```python
from build123d import *

# Parameters (mm, degrees)
BOSS_EXTRUDE1_DEPTH  = 4.7625
M4_CLEARANCE_HOLE1_D = 4.5


with BuildPart() as part:
    # Sketch1 → Boss-Extrude1 (new body)
    with BuildSketch(Plane.XY):
        with BuildLine():
            Line((288.228651321, -1867.207577199), (284.343172474, -1871.093056046))
            ThreePointArc((284.343172474, -1871.093056046), (283.201800398, -1870.89932849), (282.045921758, -1870.834481355))
            Line((282.045921758, -1870.834481355), (248.429921758, -1870.834481355))
            Line((248.429921758, -1870.834481355), (248.429921758, -1866.924781355))
            ThreePointArc((248.429921758, -1866.924781355), (242.929921758, -1861.424781355), (237.429921758, -1866.924781355))
            Line((237.429921758, -1866.924781355), (237.429921758, -1870.834481355))
            Line((237.429921758, -1870.834481355), (203.813921758, -1870.834481355))
            ThreePointArc((203.813921758, -1870.834481355), (202.658043118, -1870.89932849), (201.516671043, -1871.093056046))
            Line((201.516671043, -1871.093056046), (197.631192196, -1867.207577199))
            ThreePointArc((197.631192196, -1867.207577199), (189.853017603, -1867.207577199), (189.853017603, -1874.985751792))
            Line((189.853017603, -1874.985751792), (193.73849645, -1878.871230639))
            ThreePointArc((193.73849645, -1878.871230639), (193.544768893, -1880.012602715), (193.479921758, -1881.168481355))
            Line((193.479921758, -1881.168481355), (193.479921758, -1911.609481355))
            Line((193.479921758, -1911.609481355), (189.570221758, -1911.609481355))
            ThreePointArc((189.570221758, -1911.609481355), (184.070221758, -1917.109481355), (189.570221758, -1922.609481355))
            Line((189.570221758, -1922.609481355), (193.479921758, -1922.609481355))
            Line((193.479921758, -1922.609481355), (193.479921758, -1953.050481355))
            ThreePointArc((193.479921758, -1953.050481355), (193.544768893, -1954.206359995), (193.73849645, -1955.347732071))
            Line((193.73849645, -1955.347732071), (189.853017603, -1959.233210918))
            ThreePointArc((189.853017603, -1959.233210918), (189.853017603, -1967.011385511), (197.631192196, -1967.011385511))
            Line((197.631192196, -1967.011385511), (201.516671043, -1963.125906664))
            ThreePointArc((201.516671043, -1963.125906664), (202.658043118, -1963.31963422), (203.813921758, -1963.384481355))
            Line((203.813921758, -1963.384481355), (282.045921758, -1963.384481355))
            ThreePointArc((282.045921758, -1963.384481355), (283.201800398, -1963.31963422), (284.343172474, -1963.125906664))
            Line((284.343172474, -1963.125906664), (288.228651321, -1967.011385511))
            ThreePointArc((288.228651321, -1967.011385511), (296.006825914, -1967.011385511), (296.006825914, -1959.233210918))
            Line((296.006825914, -1959.233210918), (292.121347067, -1955.347732071))
            ThreePointArc((292.121347067, -1955.347732071), (292.315074623, -1954.206359995), (292.379921758, -1953.050481355))
            Line((292.379921758, -1953.050481355), (292.379921758, -1922.609481355))
            Line((292.379921758, -1922.609481355), (296.289621758, -1922.609481355))
            ThreePointArc((296.289621758, -1922.609481355), (301.789621758, -1917.109481355), (296.289621758, -1911.609481355))
            Line((296.289621758, -1911.609481355), (292.379921758, -1911.609481355))
            Line((292.379921758, -1911.609481355), (292.379921758, -1881.168481355))
            ThreePointArc((292.379921758, -1881.168481355), (292.315074623, -1880.012602715), (292.121347067, -1878.871230639))
            Line((292.121347067, -1878.871230639), (296.006825914, -1874.985751792))
            ThreePointArc((296.006825914, -1874.985751792), (296.006825914, -1867.207577199), (288.228651321, -1867.207577199))
        make_face()
    extrude(amount=BOSS_EXTRUDE1_DEPTH)

    # M4 Clearance Hole1 (through all)
    with Locations(Plane.XY.offset(4.7625)):
        with Locations((193.742104899, -1963.122298214), (189.570221758, -1917.109481355), (193.742104899, -1871.096664496), (242.929921758, -1866.924781355), (292.117738617, -1871.096664496), (296.289621758, -1917.109481355), (292.117738617, -1963.122298214)):
            Hole(M4_CLEARANCE_HOLE1_D / 2)


solid = part.part
```
Here's how the part is built. I have some questions about the finished solid (model axes, mm). A direction names the side the tool comes from. Round coordinates to 2 decimals unless told otherwise and drop trailing zeros. Order: outer loops, then holes, each group sorted by start corner. A loop starts at its lowest first (then second) coordinate and runs counter-clockwise, first axis right, second up. Notation, with made-up numbers: M 40,9.25 L 89,9.25 A15 cw 89,33.25 Z; hole C 4.25,86.25 d9. An arc over 180 degrees is marked long. Use CSV: the item, a comma, the result in double quotes.
1) I want a section at A-A (y = -1941). List the corners of the cut face in (x, z) for me, then the cut area to 3 significant figures.
Taken from the geometry:
outline,"M 193.48,0 L 292.38,0 L 292.38,4.76 L 193.48,4.76 Z"
area,"471 mm^2"
2) I want a section at B-B (x = 261). List the corners of the cut face in (y, z) for me, then the cut area to 3 significant figures.
Taken from the geometry:
outline,"M -1963.38,0 L -1870.83,0 L -1870.83,4.76 L -1963.38,4.76 Z"
area,"441 mm^2"
3) On a 3-axis mill with a long thin cutter (end or side, diameter ignored), from which of +Z, -Z, +X, -X, +Y, -Y can I reach the whole of each face in a straight line? I mean faces 4 (the cylindrical face through (189.768, -1966.925, 2.348)), 5 (the flat face through (192, -1911.609, 2)), 6 (the flat face through (286.313, -1869.123, 2.348)), 7 (the flat face through (294, -1911.609, 2)). Say none if no direction works.
Taken from the geometry:
face 4,"+Z, -Z"
face 5,"+Z, -Z, -X"
face 6,"+Z, -Z, +Y"
face 7,"+Z, -Z, +X"
4) I need wall thicknesses on line 1 along Y through (x, z) = (296, 3.5); line 2 along X through (y, z) = (-1872.5, 2.3); line 3 along X through (y, z) = (-1953, 4.5). Which ranges of each line are inside material? Lowest first, please. Write a range as [from, to].
Taken from the geometry:
line 1,"[-1967.02, -1959.23], [-1922.61, -1919.34], [-1914.88, -1911.61], [-1874.99, -1867.2]"
line 2,"[188.42, 191.98], [195.5, 290.36], [293.88, 297.44]"
line 3,"[193.48, 292.38]"
5) I'm going to push flat-ended pins straight in: P1, Ø2.5, axis at x = 252.5, z = 1.5, coming from the -Y side; P2, Ø1.2, axis at x = 293.5, z = 3.5, coming from the -Y side; P3, Ø1, axis at y = -1887, z = 3.5, coming from the -X side; P4, Ø4, axis at x = 193.74, y = -1963.12, coming from the +Z side (3 decimals). Where does each tip first touch, or does it pass through?
Taken from the geometry:
P1,"y = -1963.38"
P2,"y = -1968.57"
P3,"x = 193.48"
P4,"through"
6) I want a section at C-C (z = 3.75). Count the separate pieces of the cut face and the enclosed holes in it, then the cut area to 3 significant figures.
Taken from the geometry:
separate pieces,"1"
enclosed holes,"7"
area,"9,610 mm^2"
7) If we mould it in two halves opening along Y, with no side actions, what happens to faces 1 (the cylindrical face through (184.07, -1916.99, 2.35)), 2 (the flat face through (248.43, -1869, 2)), 3 (the flat face through (286.26, -1965.04, 2.35))? For each: pulls with the +Y half, pulls with the -Y half, needs draft (parallel to the pull), parting line crosses it, or undercut.
Taken from the geometry:
face 1,"undercut"
face 2,"needs draft"
face 3,"pulls with the -Y half"
